Can you work these out from the model? Positions are in its coordinate system, mm. A direction names the side the tool comes from. Give positions to 0.01 mm unless a question says otherwise; leave off trailing zeros.
from build123d import *

# Parameters (mm, degrees)
SKETCH2_W           = 110
SKETCH2_H           = 110
BOSS_EXTRUDE1_DEPTH = 8
CUT_EXTRUDE1_REACH  = 80.192
SKETCH4_R           = 1.575
SKETCH5_R           = 2.25
CUT_EXTRUDE2_DEPTH  = 3


with BuildPart() as part:
    # Sketch2 → Boss-Extrude1 (new body)
    with BuildSketch(Plane.XY):
        Rectangle(SKETCH2_W, SKETCH2_H)
    extrude(amount=BOSS_EXTRUDE1_DEPTH)

    # Sketch4 → Cut-Extrude1 (cut, up to next)
    with BuildSketch(Plane.XY.offset(8), mode=Mode.PRIVATE) as cut_extrude1_sk1:
        with Locations((-52.149125113, 52.149125113)):
            Circle(SKETCH4_R)
    cut_extrude1_tool1 = extrude(cut_extrude1_sk1.sketch, amount=-CUT_EXTRUDE1_REACH, mode=Mode.PRIVATE) & part.part
    # Sketch4 → Cut-Extrude1 (cut, up to next)
    with BuildSketch(Plane.XY.offset(8), mode=Mode.PRIVATE) as cut_extrude1_sk2:
        with Locations((-52.149125113, -52.149125113)):
            Circle(SKETCH4_R)
    cut_extrude1_tool2 = extrude(cut_extrude1_sk2.sketch, amount=-CUT_EXTRUDE1_REACH, mode=Mode.PRIVATE) & part.part
    # Sketch4 → Cut-Extrude1 (cut, up to next)
    with BuildSketch(Plane.XY.offset(8), mode=Mode.PRIVATE) as cut_extrude1_sk3:
        with Locations((52.149125113, -52.149125113)):
            Circle(SKETCH4_R)
    cut_extrude1_tool3 = extrude(cut_extrude1_sk3.sketch, amount=-CUT_EXTRUDE1_REACH, mode=Mode.PRIVATE) & part.part
    # Sketch4 → Cut-Extrude1 (cut, up to next)
    with BuildSketch(Plane.XY.offset(8), mode=Mode.PRIVATE) as cut_extrude1_sk4:
        with Locations((52.149125113, 52.149125113)):
            Circle(SKETCH4_R)
    cut_extrude1_tool4 = extrude(cut_extrude1_sk4.sketch, amount=-CUT_EXTRUDE1_REACH, mode=Mode.PRIVATE) & part.part
    add(cut_extrude1_tool1.solids().sort_by_distance((-52.149125, 52.149125, 8))[0], mode=Mode.SUBTRACT)
    add(cut_extrude1_tool2.solids().sort_by_distance((-52.149125, -52.149125, 8))[0], mode=Mode.SUBTRACT)
    add(cut_extrude1_tool3.solids().sort_by_distance((52.149125, -52.149125, 8))[0], mode=Mode.SUBTRACT)
    add(cut_extrude1_tool4.solids().sort_by_distance((52.149125, 52.149125, 8))[0], mode=Mode.SUBTRACT)

    # Sketch5 → Cut-Extrude2 (cut)
    with BuildSketch(Plane.XY.offset(8)):
        with Locations((-52.149125113, 52.149125113)):
            Circle(SKETCH5_R)
        with Locations(Location((-52.149125113, -52.149125113, 0), (0, 0, 180))):
            Circle(SKETCH5_R)
        with Locations((52.149125113, -52.149125113)):
            Circle(SKETCH5_R)
        with Locations(Location((52.149125113, 52.149125113, 0), (0, 0, 180))):
            Circle(SKETCH5_R)
    extrude(amount=-CUT_EXTRUDE2_DEPTH, mode=Mode.SUBTRACT)


solid = part.part
(1) Thinking about a two-plate mould opening in X: for faces 1 (the flat face through (-1, 55, 4)), 2 (the flat face through (55, -1, 4)), 3 (the flat face through (-54, 52, 5)), which applies, pulls with the +X half, pulls with the -X half, needs draft (parallel to the pull), parting line crosses it, or undercut?
Returned:
face 1: needs draft
face 2: pulls with the +X half
face 3: undercut
(2) Will these pins go through, and if not, where does the flat tip stop? P1, Ø3, axis at x = 52.15, y = 52.15, coming from the +Z side; P2, Ø2, axis at x = 52, y = 53, coming from the +Z side.
Returned:
P1: passes through
P2: stops at z = 5
(3) Which directions (+Z, -Z, +X, -X, +Y, -Y) give clear straight access to the entire face, cutting with the end or side of a thin tool? Please do faces 4 (the cylindrical face through (-53.723, -52.08, 2.535)), 5 (the flat face through (53, -54, 5)).
Returned:
face 4: +Z, -Z
face 5: +Z
